Build history of the part. All positions in model axes, mm. A direction names the side the tool comes from. Round coordinates to 2 decimals unless told otherwise and drop trailing zeros. Write each loop counter-clockwise with the first axis right and the second up, starting at its lowest first coordinate (ties: lowest second). Pieces come first, ordered by that corner, then holes. Notation, with made-up numbers: (62.5, -25) - (116.5, -25) arc R25 ccw to (116.5, -13) - close; hole circle Ø6 at (64, 27.25). An arc over 180 degrees is marked (long way). Write each question's results on one line, items separated by ' | '.
from build123d import *

# Parameters (mm, degrees)
BOSS_EXTRUDE1_DEPTH      = 10.16
CUT_EXTRUDE1_DEPTH       = 5.08
BOSS_EXTRUDE2_DEPTH      = 5.08
BOSS_EXTRUDE2_DEPTH_BACK = 10.16
CUT_EXTRUDE2_REACH       = 91.91
SKETCH8_W                = 23.622
SKETCH8_H                = 33.02


with BuildPart() as part:
    # Sketch1 → Boss-Extrude1 (new body)
    with BuildSketch(Plane.XY.offset(2.54)):
        with BuildLine():
            Line((-35.052, 0), (35.052, 0))
            ThreePointArc((35.052, 0), (37.207261469, 0.892738531), (38.1, 3.048))
            Line((38.1, 3.048), (38.1, 10.922))
            ThreePointArc((38.1, 10.922), (37.207261469, 13.077261469), (35.052, 13.97))
            Line((35.052, 13.97), (31.242, 13.97))
            ThreePointArc((31.242, 13.97), (29.086738531, 14.862738531), (28.194, 17.018))
            Line((28.194, 17.018), (28.194, 45.974))
            ThreePointArc((28.194, 45.974), (29.086738531, 48.129261469), (31.242, 49.022))
            Line((31.242, 49.022), (35.052, 49.022))
            ThreePointArc((35.052, 49.022), (37.207261469, 49.914738531), (38.1, 52.07))
            Line((38.1, 52.07), (38.1, 56.642))
            ThreePointArc((38.1, 56.642), (32.371594426, 70.471594426), (18.542, 76.2))
            Line((18.542, 76.2), (-18.542, 76.2))
            ThreePointArc((-18.542, 76.2), (-32.371594426, 70.471594426), (-38.1, 56.642))
            Line((-38.1, 56.642), (-38.1, 52.07))
            ThreePointArc((-38.1, 52.07), (-37.207261469, 49.914738531), (-35.052, 49.022))
            Line((-35.052, 49.022), (-31.242, 49.022))
            ThreePointArc((-31.242, 49.022), (-29.086738531, 48.129261469), (-28.194, 45.974))
            Line((-28.194, 45.974), (-28.194, 17.018))
            ThreePointArc((-28.194, 17.018), (-29.086738531, 14.862738531), (-31.242, 13.97))
            Line((-31.242, 13.97), (-35.052, 13.97))
            ThreePointArc((-35.052, 13.97), (-37.207261469, 13.077261469), (-38.1, 10.922))
            Line((-38.1, 10.922), (-38.1, 3.048))
            ThreePointArc((-38.1, 3.048), (-37.207261469, 0.892738531), (-35.052, 0))
        make_face()
    extrude(amount=-BOSS_EXTRUDE1_DEPTH)

    # Sketch2 → Cut-Extrude1 (cut)
    with BuildSketch(Plane(origin=(0, 0, -7.62), x_dir=(-1, 0, 0), z_dir=(0, 0, -1))):
        with BuildLine():
            Line((33.02, 54.102), (33.02, 56.642))
            ThreePointArc((33.02, 56.642), (28.779491978, 66.879491978), (18.542, 71.12))
            Line((18.542, 71.12), (-18.542, 71.12))
            ThreePointArc((-18.542, 71.12), (-28.779491978, 66.879491978), (-33.02, 56.642))
            Line((-33.02, 56.642), (-33.02, 54.102))
            Line((-33.02, 54.102), (-31.242, 54.102))
            ThreePointArc((-31.242, 54.102), (-25.494636083, 51.721363917), (-23.114, 45.974))
            Line((-23.114, 45.974), (-23.114, 17.018))
            ThreePointArc((-23.114, 17.018), (-25.494636083, 11.270636083), (-31.242, 8.89))
            Line((-31.242, 8.89), (-33.02, 8.89))
            Line((-33.02, 8.89), (-33.02, 5.08))
            Line((-33.02, 5.08), (33.02, 5.08))
            Line((33.02, 5.08), (33.02, 8.89))
            Line((33.02, 8.89), (31.242, 8.89))
            ThreePointArc((31.242, 8.89), (25.494636083, 11.270636083), (23.114, 17.018))
            Line((23.114, 17.018), (23.114, 45.974))
            ThreePointArc((23.114, 45.974), (25.494636083, 51.721363917), (31.242, 54.102))
            Line((31.242, 54.102), (33.02, 54.102))
        make_face()
    extrude(amount=-CUT_EXTRUDE1_DEPTH, mode=Mode.SUBTRACT)

    # Sketch7 → Boss-Extrude2 (add, two sides: drawn at the far end of the back side and taken through both)
    with BuildSketch(Plane(origin=(0, 0, -7.62), x_dir=(-1, 0, 0), z_dir=(0, 0, -1)).offset(-BOSS_EXTRUDE2_DEPTH_BACK)):
        with BuildLine():
            Line((18.542, 78.74), (-18.542, 78.74))
            ThreePointArc((-18.542, 78.74), (-34.167645651, 72.267645651), (-40.64, 56.642))
            Line((-40.64, 56.642), (-40.64, 52.07))
            ThreePointArc((-40.64, 52.07), (-39.003312693, 48.118687307), (-35.052, 46.482))
            Line((-35.052, 46.482), (-31.242, 46.482))
            ThreePointArc((-31.242, 46.482), (-30.882789755, 46.333210245), (-30.734, 45.974))
            Line((-30.734, 45.974), (-30.734, 17.018))
            ThreePointArc((-30.734, 17.018), (-30.882789755, 16.658789755), (-31.242, 16.51))
            Line((-31.242, 16.51), (-35.052, 16.51))
            ThreePointArc((-35.052, 16.51), (-39.003312693, 14.873312693), (-40.64, 10.922))
            Line((-40.64, 10.922), (-40.64, 3.048))
            ThreePointArc((-40.64, 3.048), (-39.003312693, -0.903312693), (-35.052, -2.54))
            Line((-35.052, -2.54), (35.052, -2.54))
            ThreePointArc((35.052, -2.54), (39.003312693, -0.903312693), (40.64, 3.048))
            Line((40.64, 3.048), (40.64, 10.922))
            ThreePointArc((40.64, 10.922), (39.003312693, 14.873312693), (35.052, 16.51))
            Line((35.052, 16.51), (31.242, 16.51))
            ThreePointArc((31.242, 16.51), (30.882789755, 16.658789755), (30.734, 17.018))
            Line((30.734, 17.018), (30.734, 45.974))
            ThreePointArc((30.734, 45.974), (30.882789755, 46.333210245), (31.242, 46.482))
            Line((31.242, 46.482), (35.052, 46.482))
            ThreePointArc((35.052, 46.482), (39.003312693, 48.118687307), (40.64, 52.07))
            Line((40.64, 52.07), (40.64, 56.642))
            ThreePointArc((40.64, 56.642), (34.167645651, 72.267645651), (18.542, 78.74))
        make_face()
        with BuildLine():
            ThreePointArc((-38.1, 52.07), (-37.207261469, 49.914738531), (-35.052, 49.022))
            Line((-35.052, 49.022), (-31.242, 49.022))
            ThreePointArc((-31.242, 49.022), (-29.086738531, 48.129261469), (-28.194, 45.974))
            Line((-28.194, 45.974), (-28.194, 17.018))
            ThreePointArc((-28.194, 17.018), (-29.086738531, 14.862738531), (-31.242, 13.97))
            Line((-31.242, 13.97), (-35.052, 13.97))
            ThreePointArc((-35.052, 13.97), (-37.207261469, 13.077261469), (-38.1, 10.922))
            Line((-38.1, 10.922), (-38.1, 3.048))
            ThreePointArc((-38.1, 3.048), (-37.207261469, 0.892738531), (-35.052, 0))
            Line((-35.052, 0), (35.052, 0))
            ThreePointArc((35.052, 0), (37.207261469, 0.892738531), (38.1, 3.048))
            Line((38.1, 3.048), (38.1, 10.922))
            ThreePointArc((38.1, 10.922), (37.207261469, 13.077261469), (35.052, 13.97))
            Line((35.052, 13.97), (31.242, 13.97))
            ThreePointArc((31.242, 13.97), (29.086738531, 14.862738531), (28.194, 17.018))
            Line((28.194, 17.018), (28.194, 45.974))
            ThreePointArc((28.194, 45.974), (29.086738531, 48.129261469), (31.242, 49.022))
            Line((31.242, 49.022), (35.052, 49.022))
            ThreePointArc((35.052, 49.022), (37.207261469, 49.914738531), (38.1, 52.07))
            Line((38.1, 52.07), (38.1, 56.642))
            ThreePointArc((38.1, 56.642), (32.371594426, 70.471594426), (18.542, 76.2))
            Line((18.542, 76.2), (-18.542, 76.2))
            ThreePointArc((-18.542, 76.2), (-32.371594426, 70.471594426), (-38.1, 56.642))
            Line((-38.1, 56.642), (-38.1, 52.07))
        make_face(mode=Mode.SUBTRACT)
    extrude(amount=BOSS_EXTRUDE2_DEPTH + BOSS_EXTRUDE2_DEPTH_BACK)

    # Cut-Extrude2: up to this face of the body (flat: up to its plane)
    cut_extrude2_end = Plane(part.part.faces().sort_by_distance((0, 37.604047464, 2.54))[0])
    # Sketch8 → Cut-Extrude2 (cut, up to the picked face)
    with BuildSketch(Plane(origin=(0, 0, -12.7), x_dir=(-1, 0, 0), z_dir=(0, 0, -1)), mode=Mode.PRIVATE) as cut_extrude2_sk1:
        with Locations((-34.671, 33.02)):
            Rectangle(SKETCH8_W, SKETCH8_H)
    cut_extrude2_tool1 = split(extrude(cut_extrude2_sk1.sketch, amount=-CUT_EXTRUDE2_REACH, mode=Mode.PRIVATE), bisect_by=cut_extrude2_end, keep=Keep.BOTH, mode=Mode.PRIVATE)
    # Sketch8 → Cut-Extrude2 (cut, up to the picked face)
    with BuildSketch(Plane(origin=(0, 0, -12.7), x_dir=(-1, 0, 0), z_dir=(0, 0, -1)), mode=Mode.PRIVATE) as cut_extrude2_sk2:
        with Locations((34.671, 33.02)):
            Rectangle(SKETCH8_W, SKETCH8_H)
    cut_extrude2_tool2 = split(extrude(cut_extrude2_sk2.sketch, amount=-CUT_EXTRUDE2_REACH, mode=Mode.PRIVATE), bisect_by=cut_extrude2_end, keep=Keep.BOTH, mode=Mode.PRIVATE)
    add(cut_extrude2_tool1.solids().sort_by(Axis((34.671, 33.02, -12.7), (0, 0, 1)))[0], mode=Mode.SUBTRACT)
    add(cut_extrude2_tool2.solids().sort_by(Axis((-34.671, 33.02, -12.7), (0, 0, 1)))[0], mode=Mode.SUBTRACT)


solid = part.part
(1) Flat gauge pins, fed straight in: pin 1 Ø3.5 at (x, z) = (31, -4.5) entering from +Y; pin 2 Ø4 at (y, z) = (29, 1) entering from -X; pin 3 Ø1 at (y, z) = (16.5, -1) entering from -X. Where does each tip first touch, or does it go through?
Worked answers:
pin 1: stops at y = 75.97 | pin 2: stops at x = -22.86 | pin 3: stops at x = -37.38
(2) Drill centre lines: probe 1 along Y at (x, z) = (0, -2.75); probe 2 along X at (y, z) = (4.5, -11); probe 3 along Y at (x, z) = (-12, -9.25). Where is each one in solid material? Low to high. Write a range as [from, to].
Worked answers:
probe 1: y = [-2.54, 5.08], [71.12, 78.74] | probe 2: x = [-40.64, -38.1], [38.1, 40.64] | probe 3: y = [-2.54, 0], [76.2, 78.74]
(3) Slice it at C-C, the plane y = 63. Write the cut outline in (x, z).
Worked answers:
outline: (-39.71, -12.7) - (-37.04, -12.7) - (-37.04, -7.62) - (-31.55, -7.62) - (-31.55, -2.54) - (31.55, -2.54) - (31.55, -7.62) - (37.04, -7.62) - (37.04, -12.7) - (39.71, -12.7) - (39.71, 2.54) - (-39.71, 2.54) - close
(4) Slice it at D-D, the plane y = 30.5. Write the cut outline in (x, z).
Worked answers:
outline: (-22.86, -2.54) - (22.86, -2.54) - (22.86, 2.54) - (-22.86, 2.54) - close
(5) Slice it at B-B, the plane x = -6. Write the cut outline in (y, z).
Worked answers:
outline: (-2.54, -12.7) - (0, -12.7) - (0, -7.62) - (5.08, -7.62) - (5.08, -2.54) - (71.12, -2.54) - (71.12, -7.62) - (76.2, -7.62) - (76.2, -12.7) - (78.74, -12.7) - (78.74, 2.54) - (-2.54, 2.54) - close
(6) Tool access for faces 4 (the flat face through (-29, 16.51, -3)), 5 (the cylindrical face through (40.49, 50.78, -4.97)), 6 (the flat face through (-3, 72, -7.62)): list every direction of +Z, -Z, +X, -X, +Y, -Y with a clear straight run to the whole face (end or side of a thin tool).
Worked answers:
face 4: +Z, -Z, -X | face 5: +Z, -Z, +X | face 6: -Z
(7) Two-plate mould, pull along Y, no slides. Class faces 1 (the cylindrical face through (-38.96, -0.947, -4.973)), 2 (the flat face through (0, 78.74, -5)), 3 (the flat face through (33, 13.97, -10)): released by +Y, released by -Y, zero draft, split by the parting line, or undercut.
Worked answers:
face 1: released by -Y | face 2: released by +Y | face 3: undercut
